Autodesk Inventor part; units mm, degrees
ref_plane "YZ Plane" through (0, 0, 0) normal (1, 0, 0) x (0, 1, 0)
ref_plane "XZ Plane" through (0, 0, 0) normal (0, 1, 0) x (-1, 0, 0)
ref_plane "XY Plane" through (0, 0, 0) normal (0, 0, 1) x (1, 0, 0)
sketch "Sketch1" plane through (0, 0, 0) normal (0, 1, 0) x (-1, 0, 0)
  line L0 (0, 0) -> (-76.2, 0)
  line L1 (-76.2, 0) -> (-76.2, -63.5) construction
  line L2 (-76.2, -63.5) -> (0, -63.5)
  line L3 (0, -63.5) -> (0, 0) construction
  line L4 (0, -31.75) -> (44.45, -31.75) construction
  line L5 (-76.2, -31.75) -> (-127, -31.75) construction
  circle A0 centre (44.45, -31.75) radius 3.175
  circle A1 centre (-127, -31.75) radius 3.175 construction
  circle A2 centre (-114.3, -31.75) radius 3.175 construction
  line L6 (-114.3, -34.925) -> (-127, -34.925)
  line L7 (-114.3, -28.575) -> (-127, -28.575)
  arc A3 (-114.3, -34.925) -> (-114.3, -28.575) centre (-114.3, -31.75) ccw
  arc A4 (-127, -28.575) -> (-127, -34.925) centre (-127, -31.75) ccw
  line L8 (0, -63.5) -> (47.5152, -37.3112)
  line L9 (47.5152, -26.1888) -> (0, 0)
  line L10 (-76.2, -63.5) -> (-129.7757, -37.4612)
  line L11 (-129.7757, -26.0388) -> (-76.2, 0)
  arc A5 (47.5152, -37.3112) -> (47.5152, -26.1888) centre (44.45, -31.75) ccw
  arc A6 (-129.7757, -26.0388) -> (-129.7757, -37.4612) centre (-127, -31.75) ccw
  circle A7 centre (-76.2, -31.75) radius 3.175 construction
  circle A8 centre (-63.5, -31.75) radius 3.175 construction
  line L12 (-76.2, -28.575) -> (-63.5, -28.575) construction
  line L13 (-76.2, -34.925) -> (-63.5, -34.925) construction
  line L14 (-63.5, -28.575) -> (-76.2, -28.575)
  line L15 (-76.2, -34.925) -> (-63.5, -34.925)
  arc A9 (-63.5, -34.925) -> (-63.5, -28.575) centre (-63.5, -31.75) ccw
  arc A10 (-76.2, -28.575) -> (-76.2, -34.925) centre (-76.2, -31.75) ccw
  circle A11 centre (0, -31.75) radius 3.175 construction
  circle A12 centre (-12.7, -31.75) radius 3.175 construction
  line L16 (0, -28.575) -> (-12.7, -28.575) construction
  line L17 (0, -34.925) -> (-12.7, -34.925) construction
  arc A13 (-12.7, -28.575) -> (-12.7, -34.925) centre (-12.7, -31.75) ccw
  arc A14 (0, -34.925) -> (0, -28.575) centre (0, -31.75) ccw
  line L18 (-12.7, -34.925) -> (0, -34.925)
  line L19 (-12.7, -28.575) -> (0, -28.575)
  dimension "d0" = 76.2
  dimension "d1" = 63.5
  dimension "d2" = 44.45
  dimension "d3" = 50.8
  dimension "d4" = 6.35
  dimension "d5" = 6.35
  dimension "d6" = 6.35
  dimension "d7" = 12.7
  dimension "d8" = 6.35
  dimension "d9" = 0
  dimension "d10" = 0
  dimension "d11" = 0
  dimension "d12" = 0
  dimension "d13" = 6.35
  dimension "d14" = 6.35
  dimension "d15" = 12.7
  dimension "d16" = 0
  dimension "d17" = 6.35
  dimension "d18" = 6.35
  dimension "d19" = 0
  dimension "d20" = 12.7
extrude "Extrusion1" add sketch "Sketch1" along normal blind 3.175
sketch "Sketch2" plane through (0, 0, 0) normal (0, 0, 1) x (1, 0, 0)
  line L0 (0, 0) -> (76.2, 0)
  line L1 (76.2, 0) -> (76.2, 3.175)
  line L2 (0, 3.175) -> (76.2, 3.175)
  line L3 (0, 0) -> (0, 3.175)
  circle A0 centre (25.4, 28.575) radius 5.5562
  circle A1 centre (44.45, 19.05) radius 5.5563
  line L4 (0, 3.175) -> (17.12, 33.2832)
  line L5 (29.6597, 37.0944) -> (48.7097, 27.5694)
  line L6 (50.8395, 26.114) -> (76.2, 3.175)
  arc A2 (29.6597, 37.0944) -> (17.12, 33.2832) centre (25.4, 28.575) ccw
  arc A3 (50.8395, 26.114) -> (48.7097, 27.5694) centre (44.45, 19.05) ccw
  dimension "d23" = 11.1125
  dimension "d24" = 28.575
  dimension "d25" = 25.4
  dimension "d26" = 11.1125
  dimension "d27" = 19.05
  dimension "d28" = 31.75
  dimension "d29" = 9.525
extrude "Extrusion2" add sketch "Sketch2" against normal blind 3.175
sketch "Sketch3" plane through (76.2, 0, -63.5) normal (0, 0, -1) x (-1, 0, 0)
  line L0 (0, 0) -> (76.2, 0)
  line L1 (76.2, 0) -> (76.2, 3.175)
  line L2 (0, 3.175) -> (76.2, 3.175)
  line L3 (0, 0) -> (0, 3.175)
  line L4 (76.2, 3.175) -> (0, 3.175)
  line L5 (76.2, 3.175) -> (59.08, 33.2832)
  arc A0 (59.08, 33.2832) -> (46.5403, 37.0944) centre (50.8, 28.575) ccw
  line L6 (46.5403, 37.0944) -> (27.4903, 27.5694)
  arc A1 (27.4903, 27.5694) -> (25.3605, 26.114) centre (31.75, 19.05) ccw
  line L7 (25.3605, 26.114) -> (0, 3.175)
  circle A2 centre (31.75, 19.05) radius 5.5563
  circle A3 centre (50.8, 28.575) radius 5.5562
  point P0 (76.2, 0)
extrude "Extrusion3" add sketch "Sketch3" against normal blind 3.175
sketch "Sketch4" plane through (0, 0, 0) normal (0, 0, 1) x (1, 0, 0)
  circle A0 centre (44.45, 19.05) radius 5.5563
  circle A1 centre (25.4, 28.575) radius 5.5562
  line L0 (0, 0) -> (76.2, 0)
  line L1 (76.2, 0) -> (76.2, 3.175)
  line L2 (76.2, 3.175) -> (50.8395, 26.114)
  arc A2 (50.8395, 26.114) -> (48.7097, 27.5694) centre (44.45, 19.05) ccw
  line L3 (48.7097, 27.5694) -> (29.6597, 37.0944)
  arc A3 (29.6597, 37.0944) -> (17.12, 33.2832) centre (25.4, 28.575) ccw
  line L4 (17.12, 33.2832) -> (0, 3.175)
  line L5 (0, 0) -> (0, 3.175)
  circle A4 centre (25.4, 28.575) radius 4.7625
  circle A5 centre (44.45, 19.05) radius 4.7625
  dimension "d34" = 9.525
  dimension "d35" = 9.525
extrude "Extrusion4" add sketch "Sketch4" against normal blind 63.5 contours A0 | A1
properties part number "garage door hinge"
For this review, take the finished solid that the model builds, in its own axes (mm). A direction names the side the tool comes from. Coordinates: 2 decimals unless noted, no trailing zeros. Write each loop counter-clockwise with the first axis right and the second up, starting at its lowest first coordinate (ties: lowest second). Pieces come first, ordered by that corner, then holes. Notation, with made-up numbers: (70, -13.75) -> (121, -13.75) arc R22 cw to (121, 8.25) -> close; hole circle Ø7 at (61.5, 33.25). An arc over 180 degrees is marked (long way). Put each result on its own line as item: value.
Q1. Tool access review of faces 1 (the cylindrical face through (27.964, 23.646, -31.35)), 2 (the cylindrical face through (-3.174, 1.565, -31.68)), 3 (the flat face through (-23.42, 1.57, -50.59)): name each direction out of +Z, -Z, +X, -X, +Y, -Y from which nothing blocks a thin tool from reaching the whole face with its end or side.
From the geometry:
face 1: none
face 2: +Y, -Y
face 3: -Z, -X, +Y, -Y
Q2. Take a section at A-A, the plane x = 25.4. State the section outline as (y, z) points (1 decimal).
From the geometry:
outline: (0, -63.5) -> (23.8, -63.5) -> (23.8, 0) -> (0, 0) -> close; (33.3, -63.5) -> (38.1, -63.5) -> (38.1, -60.3) -> (34.1, -60.3) -> (34.1, -3.2) -> (38.1, -3.2) -> (38.1, 0) -> (33.3, 0) -> close; hole (3.2, -60.3) -> (23, -60.3) -> (23, -3.2) -> (3.2, -3.2) -> close
Q3. Take a section at D-D, the plane y = 19.05. State the section outline as (x, z) points (1 decimal).
From the geometry:
outline: (9, -63.5) -> (39.7, -63.5) -> (39.7, 0) -> (9, 0) -> (9, -3.2) -> (38.9, -3.2) -> (38.9, -60.3) -> (9, -60.3) -> close; (49.2, -63.5) -> (58.6, -63.5) -> (58.6, -60.3) -> (50, -60.3) -> (50, -3.2) -> (58.6, -3.2) -> (58.6, 0) -> (49.2, 0) -> close
Q4. Take a section at B-B, the plane z = -13. Count the separate pieces of the cut face and the enclosed holes in it, then the cut area to 3 significant figures.
From the geometry:
separate pieces: 3
enclosed holes: 2
area: 453 mm2
Q5. Wall thickness on L1, parallel to Y at x = 25.4, z = -44 (1 decimal); L2, parallel to Y at x = 44.45, z = -34.5 (1 decimal); L3, parallel to Z at x = 56.5, y = 8.5 (3 decimals): over which ranges is each line inside the solid? List them lowest first.
From the geometry:
L1: y = 0 to 3.2, 23 to 23.8, 33.3 to 34.1
L2: y = 0 to 3.2, 13.5 to 14.3, 23.8 to 24.6
L3: z = -63.5 to -60.325, -3.175 to 0
Q6. Clearance check with flat-ended pins moving along their axes: pin 1 Ø3 at (x, z) = (-6.5, -52.5) entering from +Y (3 decimals); pin 2 Ø1 at (y, z) = (22, -17.5) entering from +X; pin 3 Ø1.6 at (x, y) = (118, 2.5) entering from -Z; pin 4 Ø5 at (x, z) = (-44.45, -31.75) entering from +Y. State where each tip first meets the part, or that it passes through.
From the geometry:
pin 1: stops at y = 3.175
pin 2: stops at x = 49.44
pin 3: stops at z = -43.57
pin 4: passes through
Q7. The part is to be moulded in two halves that separate along X. For faces 4 (the cylindrical face through (-43.76, 1.57, -28.65)), 5 (the cylindrical face through (-50.8, 1.6, -31.7)), 6 (the cylindrical face through (22.73, 37.72, -1.57)), say which applies: +X half, -X half, draft (parallel to the pull), parting line (faces both ways), or undercut.
From the geometry:
face 4: undercut
face 5: -X half
face 6: parting line
